```python
from build123d import *

# Parameters (mm, degrees)
SKETCH2_R               = 15.5
SKETCH2_R_2             = 14
BOSS_EXTRUDE1_DEPTH     = 20
SKETCH3_OUTSIDE_W       = 42.638
SKETCH3_OUTSIDE_H       = 42.638
CUT_EXTRUDE1_DEPTH      = 21
SKETCH6_R               = 2
BOSS_EXTRUDE2_DEPTH     = 1.5
CUT_EXTRUDE4_DEPTH      = 21
CUT_EXTRUDE4_DEPTH_BACK = 10
SKETCH9_R               = 2.5
CUT_EXTRUDE5_DEPTH      = 10
FILLET1_R               = 3


with BuildPart() as part:
    # Sketch2 → Boss-Extrude1 (new body)
    with BuildSketch(Plane(origin=(0, 0, 0), x_dir=(1, 0, 0), z_dir=(0, 1, 0))):
        Circle(SKETCH2_R)
        Circle(SKETCH2_R_2, mode=Mode.SUBTRACT)
    boss_extrude1 = extrude(amount=BOSS_EXTRUDE1_DEPTH)

    # Sketch3 outside → Cut-Extrude1 (cut, through all)
    with BuildSketch(Plane(origin=(0, 20, 0), x_dir=(1, 0, 0), z_dir=(0, 1, 0))):
        Rectangle(SKETCH3_OUTSIDE_W, SKETCH3_OUTSIDE_H)
        with BuildLine():
            Line((0, 0), (7.5, 13.564659966))
            ThreePointArc((7.5, 13.564659966), (0, 15.5), (-7.5, 13.564659966))
            Line((-7.5, 13.564659966), (0, 0))
        make_face(mode=Mode.SUBTRACT)
    extrude(amount=-CUT_EXTRUDE1_DEPTH, mode=Mode.SUBTRACT)

    # Sketch6 → Boss-Extrude2 (add, symmetric)
    with BuildSketch(Plane(origin=(0, 7.5, 0), x_dir=(0, 1, 0), z_dir=(-1, 0, 0))):
        with BuildLine():
            Line((-0.5, 20.5), (-0.5, 15.25))
            Line((-0.5, 15.25), (5.5, 15.25))
            Line((5.5, 15.25), (5.5, 20.5))
            ThreePointArc((5.5, 20.5), (2.5, 23.5), (-0.5, 20.5))
        make_face()
        with Locations((2.5, 20.5)):
            Circle(SKETCH6_R, mode=Mode.SUBTRACT)
    boss_extrude2 = extrude(amount=BOSS_EXTRUDE2_DEPTH, both=True)

    # Mirror2: Boss-Extrude1, Boss-Extrude2 across plane
    add(boss_extrude1.mirror(Plane(origin=(0, 0, 0), x_dir=(-0.483870968, 0, 0.875139353), z_dir=(0.875139353, 0, 0.483870968))))
    add(boss_extrude2.mirror(Plane(origin=(0, 0, 0), x_dir=(-0.483870968, 0, 0.875139353), z_dir=(0.875139353, 0, 0.483870968))))

    # Sketch8 → Cut-Extrude4 (cut, two sides)
    with BuildSketch(Plane(origin=(0, 0, 0), x_dir=(1, 0, 0), z_dir=(0, 1, 0))) as cut_extrude4_sk:
        with BuildLine():
            Line((-5.570225317, 14.464528679), (0, 0))
            Line((0, 0), (15.212039463, 2.973862033))
            ThreePointArc((15.212039463, 2.973862033), (-7.5, -13.564659966), (-5.570225317, 14.464528679))
        make_face()
    extrude(amount=CUT_EXTRUDE4_DEPTH, mode=Mode.SUBTRACT)
    extrude(cut_extrude4_sk.sketch, amount=-CUT_EXTRUDE4_DEPTH_BACK, mode=Mode.SUBTRACT)

    # Sketch9 → Cut-Extrude5 (cut)
    with BuildSketch(Plane(origin=(4.354367679, 0, -7.875402257), x_dir=(-0.875139353, 0, -0.483870968), z_dir=(0.483870968, 0, -0.875139353))):
        with Locations((0, 15)):
            Circle(SKETCH9_R)
        with Locations((0, 5)):
            Circle(SKETCH9_R)
    extrude(amount=CUT_EXTRUDE5_DEPTH, mode=Mode.SUBTRACT)

    # Fillet1
    fillet1_edges = [part.edges().sort_by_distance(p)[0] for p in [
        (-1.5, 10, -15.427248621),
        (1.5, 10, -15.427248621),
        (13.863083148, 10, -6.932887251),
        (12.267869828, 10, -9.473614404),
    ]]
    fillet(fillet1_edges, radius=FILLET1_R)


solid = part.part
```
Work out the finished part from the listing and answer in its coordinate system (mm). A direction names the side the tool comes from. Give positions to 0.01 mm unless a question says otherwise; leave off trailing zeros. Loops run counter-clockwise (first coordinate to the right, second up) from the corner with the lowest first, then second, coordinate; pieces in that order, holes last. Notation, with made-up numbers: (-32.75, 48) -> (-3.75, 48) arc R9 ccw to (-3.75, 64) -> close; hole circle Ø6 at (-0.75, 11.5). An arc over 180 degrees is marked (long way). Use CSV: the item, a comma, the result in double quotes.
1. The mould has two halves that part along X. Classify faces 1 (the cylindrical face through (2.15, 9.96, -16.08)), 2 (the cylindrical face through (0, 10.1, -23.5)), 3 (the cylindrical face through (5.054, 14.042, -13.914)): +X half, -X half, draft (parallel to the pull), parting line (faces both ways), or undercut.
Found:
face 1,"+X half"
face 2,"draft"
face 3,"undercut"
2. Straight lines are drawn through the part: line 1 (Z direction, x = 0.15, y = 10); line 2 (Y direction, x = -0.5, z = -20.5); line 3 (X direction, y = 11, z = -12). For each, find the intervals that lie inside material, in ascending order.
Found:
line 1,"-23.5 to -22.5, -18.5 to -14"
line 2,"7 to 8, 12 to 13"
line 3,"7.21 to 9.81, 18.72 to 20.01"
3. A tool of negligible diameter and unlimited length cuts with its end or side. For faces 4 (the flat face through (15.74, 7.958, -11.653)), 5 (the flat face through (1.5, 8, -19.5)), 6 (the flat face through (-1.5, 8, -19.5)), from which of +Z, -Z, +X, -X, +Y, -Y can it reach the whole face along a straight path? Write none if from no direction.
Found:
face 4,"-Z, +Y, -Y"
face 5,"-Z, +X, +Y, -Y"
face 6,"-Z, -X, +Y, -Y"
4. The part is cut by section B-B (z = -19.25). Write down the section's boundary in (x, y), then the cut area to 3 significant figures.
Found:
outline,"(-1.5, 7) -> (1.5, 7) -> (1.5, 8.44) -> (-1.5, 8.44) -> close; (-1.5, 11.56) -> (1.5, 11.56) -> (1.5, 13) -> (-1.5, 13) -> close"
area,"8.63 mm^2"
5. The part is cut by section C-C (y = 10). Write down the section's boundary in (x, z).
Found:
outline,"(-5.57, -14.46) arc R15.5 ccw to (-3.77, -15.03) arc R3 cw to (-1.5, -17.94) -> (-1.5, -18.5) -> (1.5, -18.5) -> (1.5, -17.94) arc R3 cw to (3.77, -15.03) arc R15.5 ccw to (10.73, -11.19) arc R3 cw to (14.4, -10.81) -> (14.87, -11.11) -> (16.47, -8.57) -> (15.99, -8.27) arc R3 cw to (14.74, -4.8) arc R15.5 ccw to (15.21, -2.97) -> (13.74, -2.69) arc R14 cw to (-5.03, -13.06) -> close; (-1.5, -23.5) -> (1.5, -23.5) -> (1.5, -22.5) -> (-1.5, -22.5) -> close; (18.26, -13.23) -> (19.1, -13.77) -> (20.7, -11.23) -> (19.85, -10.69) -> close"
6. The part is cut by section A-A (y = 4). Write down the section's boundary in (x, z).
Found:
outline,"(-5.57, -14.46) arc R15.5 ccw to (5.41, -14.52) -> (4.68, -13.2) arc R14 cw to (-5.03, -13.06) -> close; (8.69, -10.98) -> (9.42, -12.31) arc R15.5 ccw to (15.21, -2.97) -> (13.74, -2.69) arc R14 cw to start"
7. The part is cut by section D-D (y = 18.25). Write down the section's boundary in (x, z).
Found:
outline,"(-5.57, -14.46) arc R15.5 ccw to (15.21, -2.97) -> (13.74, -2.69) arc R14 cw to (-5.03, -13.06) -> close"
8. Flat-ended cylindrical pins translate along their axes: pin 1 Ø3 at (y, z) = (10, -19.5) entering from +X; pin 2 Ø10 at (x, z) = (3, -5.5) entering from -Y; pin 3 Ø1.6 at (x, z) = (-1.5, -18.5) entering from -Y; pin 4 Ø4.5 at (x, z) = (-1, -18.5) entering from +Y. Find the tip coordinate at first contact, or state that the pin passes through.
Found:
pin 1,"x = 1.5"
pin 2,"through"
pin 3,"y = 7"
pin 4,"y = 13"
